Verification items for the finished model (mm, model axes). A direction names the side the tool comes from. Coordinates: 2 decimals unless noted, no trailing zeros. Order: outer loops, then holes, each group sorted by start corner. A loop starts at its lowest first (then second) coordinate and runs counter-clockwise, first axis right, second up. Notation, with made-up numbers: M -19.75,31 L 27.25,31 A18 cw 27.25,60 Z; hole C 36.5,22.25 d4. An arc over 180 degrees is marked long. Return JSON: item names as keys, results as strings. Group by question number.
1. Section check D-D, the plane x = -14. Record the cut outline in (y, z).
2. Section check A-A, the plane z = 1.1. Record the cut outline in (x, y), plus the area to 3 significant figures.
3. Section check C-C, the plane y = 7.25. Record the cut outline in (x, z), plus the area to 3 significant figures.
4. Gauge pin test, flat ends, axial feed: pin 1 (1.2 mm diameter, centred on y = 4.5, z = 2, fed in from +X); pin 2 (2 mm diameter, centred on x = 17.5, y = 0, fed in from +Z); pin 3 (6 mm diameter, centred on x = -6, y = 2, fed in from -Z); pin 4 (1 mm diameter, centred on x = -6.5, z = 1.5, fed in from +Y). Record the tip position at first contact, or that the pin passes through.
5. Section check B-B, the plane x = 9. Record the cut outline in (y, z).
6. Set-up check for faces 5 (the flat face through (-16, 2.75, 1)), 6 (the flat face through (16, -2.75, 1)), 7 (the cylindrical face through (-9, -6, 2)): record each of +Z, -Z, +X, -X, +Y, -Y from which the full face is reachable in a straight line by a thin tool's end or side.
7. Mould release check, pull along Y, two halves, no side actions. Record for faces 1 (the flat face through (4.2, 0.2, 3)), 2 (the flat face through (-16, -2.75, 1)), 3 (the cylindrical face through (-20.25, -0.06, 1.48)), 4 (the flat face through (1, 0, 2)): +Y half, -Y half, draft (parallel to the pull), parting line (faces both ways), or undercut.
8. Material ranges on line 1 along Y through (x, z) = (17.5, 1.9); line 2 along X through (y, z) = (10, 1.6), recorded low to high.
Autodesk Inventor part; units mm, degrees
ref_plane "YZ Plane" through (0, 0, 0) normal (1, 0, 0) x (0, 1, 0)
ref_plane "XZ Plane" through (0, 0, 0) normal (0, 1, 0) x (-1, 0, 0)
ref_plane "XY Plane" through (0, 0, 0) normal (0, 0, 1) x (1, 0, 0)
sketch "스케치1" plane through (0, 0, 0) normal (0, 0, 1) x (1, 0, 0)
  circle A0 centre (0, 0) radius 13.75
  circle A1 centre (17.5, 0) radius 1.25
  circle A2 centre (17.5, 0) radius 2.75
  line L0 (17.5, 2.75) -> (13.4722, 2.75)
  line L1 (17.5, -2.75) -> (13.4722, -2.75)
  line L2 (0, 0) -> (0, 3.2191)
  circle A3 centre (-17.5, 0) radius 1.25
  circle A4 centre (-17.5, 0) radius 2.75
  line L3 (-17.5, 2.75) -> (-13.4722, 2.75)
  line L4 (-17.5, -2.75) -> (-13.4722, -2.75)
  dimension "d0" = 27.5
  dimension "d1" = 2.5
  dimension "d2" = 5.5
  dimension "d22" = 35
extrude "돌출1" add sketch "스케치1" along normal blind 3
sketch "스케치2" plane through (0, 0, 0) normal (0, 0, -1) x (-1, 0, 0)
  circle A0 centre (0, 0) radius 12
  dimension "d5" = 24
extrude "돌출2" cut sketch "스케치2" against normal blind 1.5
sketch "스케치3" plane through (0, 0, 1.5) normal (0, 0, -1) x (-1, 0, 0)
  line L0 (0, 10.5) -> (0, -10.5) construction
  line L1 (-1, 10.5) -> (-1, -10.5)
  line L2 (1, -10.5) -> (1, 10.5)
  arc A0 (1, 10.5) -> (-1, 10.5) centre (0, 10.5) ccw
  arc A1 (-1, -10.5) -> (1, -10.5) centre (0, -10.5) ccw
  line L3 (3, -10) -> (3, 10) construction
  line L4 (4, -10) -> (4, 10)
  line L5 (2, 10) -> (2, -10)
  arc A2 (2, -10) -> (4, -10) centre (3, -10) ccw
  arc A3 (4, 10) -> (2, 10) centre (3, 10) ccw
  line L6 (6, -8.5) -> (6, 8.5) construction
  line L7 (7, -8.5) -> (7, 8.5)
  line L8 (5, 8.5) -> (5, -8.5)
  arc A4 (5, -8.5) -> (7, -8.5) centre (6, -8.5) ccw
  arc A5 (7, 8.5) -> (5, 8.5) centre (6, 8.5) ccw
  line L9 (9, -5) -> (9, 5) construction
  line L10 (10, -5) -> (10, 5)
  line L11 (8, 5) -> (8, -5)
  arc A6 (8, -5) -> (10, -5) centre (9, -5) ccw
  arc A7 (10, 5) -> (8, 5) centre (9, 5) ccw
  line L12 (-3, -10) -> (-3, 10) construction
  line L13 (-4, -10) -> (-4, 10)
  line L14 (-2, 10) -> (-2, -10)
  arc A8 (-4, -10) -> (-2, -10) centre (-3, -10) ccw
  arc A9 (-2, 10) -> (-4, 10) centre (-3, 10) ccw
  line L15 (-6, -8.5) -> (-6, 8.5) construction
  line L16 (-7, -8.5) -> (-7, 8.5)
  line L17 (-5, 8.5) -> (-5, -8.5)
  arc A10 (-7, -8.5) -> (-5, -8.5) centre (-6, -8.5) ccw
  arc A11 (-5, 8.5) -> (-7, 8.5) centre (-6, 8.5) ccw
  line L18 (-9, -5) -> (-9, 5) construction
  line L19 (-10, -5) -> (-10, 5)
  line L20 (-8, 5) -> (-8, -5)
  arc A12 (-10, -5) -> (-8, -5) centre (-9, -5) ccw
  arc A13 (-8, 5) -> (-10, 5) centre (-9, 5) ccw
  point P0 (0, 0)
  point P1 (3, 0)
  point P2 (6, 0)
  point P3 (9, 0)
  point P4 (-3, 0)
  point P5 (-6, 0)
  point P6 (-9, 0)
  dimension "d8" = 21
  dimension "d9" = 1
  dimension "d10" = 1
  dimension "d11" = 1
  dimension "d12" = 20
  dimension "d13" = 17
  dimension "d14" = 1
  dimension "d15" = 1
  dimension "d17" = 1
  dimension "d18" = 10
  dimension "d19" = 1
extrude "돌출3" cut sketch "스케치3" against normal blind 1.5
properties part number "스피커 홀더"
Answers follow:
{
 "1": {"outline": "M -2.75,0 L 2.75,0 L 2.75,3 L -2.75,3 Z"},
 "2": {"outline": "M -17.5,-2.75 L -13.47,-2.75 A13.75 ccw 13.47,-2.75 L 17.5,-2.75 A2.75 ccw 17.5,2.75 L 13.47,2.75 A13.75 ccw -13.47,2.75 L -17.5,2.75 A2.75 ccw Z; hole C -17.5,0 d2.5; hole C 0,0 d24; hole C 17.5,0 d2.5", "area": "198 mm^2"},
 "3": {"outline": "M -11.68,0 L -9.56,0 L -9.56,1.5 L -7,1.5 L -7,3 L -11.68,3 Z; M -5,1.5 L -4,1.5 L -4,3 L -5,3 Z; M -2,1.5 L -1,1.5 L -1,3 L -2,3 Z; M 1,1.5 L 2,1.5 L 2,3 L 1,3 Z; M 4,1.5 L 5,1.5 L 5,3 L 4,3 Z; M 7,1.5 L 9.56,1.5 L 9.56,0 L 11.68,0 L 11.68,3 L 7,3 Z", "area": "26.4 mm^2"},
 "4": {"pin 1": "x = 13.19", "pin 2": "through", "pin 3": "z = 1.5", "pin 4": "y = 12.37"},
 "5": {"outline": "M -10.4,0 L -7.94,0 L -7.94,1.5 L -6,1.5 L -6,3 L -10.4,3 Z; M 6,1.5 L 7.94,1.5 L 7.94,0 L 10.4,0 L 10.4,3 L 6,3 Z"},
 "6": {"face 5": "+Z, -Z, -X, +Y", "face 6": "+Z, -Z, +X, -Y", "face 7": "+Z, -Z"},
 "7": {"face 1": "draft", "face 2": "-Y half", "face 3": "parting line", "face 4": "undercut"},
 "8": {"line 1": "-2.75 to -1.25, 1.25 to 2.75", "line 2": "-9.44 to -4, -2 to -1, 1 to 2, 4 to 9.44"}
}
